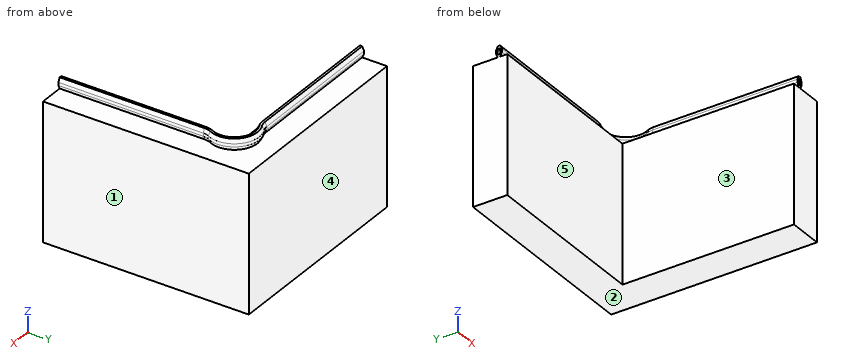
from build123d import *

# Parameters (mm, degrees)
F1_DEPTH = 100


with BuildPart() as f1:
    # F0 (on Top) → F1 (new body)
    with BuildSketch(Plane.XY):
        Polygon((0, -150), (0, 0), (-150, 0), (-150, -25), (-25, -25), (-25, -150), align=None)
    extrude(amount=F1_DEPTH)

    # F4: sweep along a path in F2
    with BuildLine(Plane.XY.offset(100)) as f4_path:
        Line((-150, -18.9), (-44.4089054678, -18.9))
        ThreePointArc((-44.4089054678, -18.9), (-41.6782966505, -18.5851947133), (-39.0909561818, -17.6572959145))
        ThreePointArc((-39.0909561818, -17.6572959145), (-20.6866486348, -20.6866486348), (-17.6572959145, -39.0909561818))
        ThreePointArc((-17.6572959145, -39.0909561818), (-18.5851947133, -41.6782966505), (-18.9, -44.4089054678))
        Line((-18.9, -44.4089054678), (-18.9, -150))
    # F3 (on face) → F4 (sweep)
    with BuildSketch(Plane(origin=(-150, 0, 0), x_dir=(0, -1, 0), z_dir=(-1, 0, 0))):
        Polygon((16.7, 102.875), (18.0713046565, 100), (19.7286953435, 100), (21.1, 102.875), (21.1, 105.075), (19.7286953435, 107.95), (18.0713046565, 107.95), (16.7, 105.075), align=None)
        Polygon((17.75, 104.971631851), (18.2285820574, 105.975), (19.5714179426, 105.975), (20.05, 104.971631851), (20.05, 102.978368149), (19.5714179426, 101.975), (18.2285820574, 101.975), (17.75, 102.978368149), align=None, mode=Mode.SUBTRACT)
    sweep(path=f4_path.line)


solid = f1.part
Work out the finished part from the listing and answer in its coordinate system (mm). Face numbers are marked on the shaded views. A direction names the side the tool comes from. Coordinates: 2 decimals unless noted, no trailing zeros. Write each loop counter-clockwise with the first axis right and the second up, starting at its lowest first coordinate (ties: lowest second). Pieces come first, ordered by that corner, then holes. Notation, with made-up numbers: (6.5, 73.5) - (59.5, 73.5) arc R24 ccw to (59.5, 108.5) - close; hole circle Ø7 at (27, 75). An arc over 180 degrees is marked (long way). One line per question, with ' | ' between items.
1) Find section A-A, the plane y = -69.5. Determine the outline of the cut face in (x, z) (3 decimals).
Checks:
outline: (-25, 0) - (0, 0) - (0, 100) - (-18.071, 100) - (-16.7, 102.875) - (-16.7, 105.075) - (-18.071, 107.95) - (-19.729, 107.95) - (-21.1, 105.075) - (-21.1, 102.875) - (-19.729, 100) - (-25, 100) - close; hole (-20.05, 102.978) - (-19.571, 101.975) - (-18.229, 101.975) - (-17.75, 102.978) - (-17.75, 104.972) - (-18.229, 105.975) - (-19.571, 105.975) - (-20.05, 104.972) - close
2) For the marked faces 4 and 5, determine the directions among +Z, -Z, +X, -X, +Y, -Y from which every point of the face is accessible in a straight line to the end or side of a thin tool.
Checks:
face 4: +Z, -Z, +X, -X, +Y | face 5: +Z, -Z, -X, -Y
3) Find section D-D, the plane x = -9.5. Determine the outline of the cut face in (y, z), and give its area (3 significant figures).
Checks:
outline: (-150, 0) - (0, 0) - (0, 100) - (-150, 100) - close | area: 15,000 mm2
4) Flat-ended cylindrical pins translate along their axes: P1, Ø0.6, axis at y = -98, z = 104, coming from the -X side; P2, Ø2, axis at y = -85, z = 67.5, coming from the -X side; P3, Ø2, axis at x = -128, z = 53.5, coming from the -Y side. Find the tip coordinate at first contact, or state that the pin passes through.
Checks:
P1: x = -21.1 | P2: x = -25 | P3: y = -25
5) The mould has two halves that part along X. Classify the marked faces 1, 2 and 3: +X half, -X half, draft (parallel to the pull), parting line (faces both ways), or undercut.
Checks:
face 1: +X half | face 2: draft | face 3: -X half
6) Consider probe 1 along X at (y, z) = (-121, 77.5); probe 2 along X at (y, z) = (-86, 102.5). Determine where each line is inside the solid, lowest interval first. Write a range as [from, to].
Checks:
probe 1: [-25, 0] | probe 2: [-20.92, -19.82], [-17.98, -16.88]
7) Find section C-C, the plane z = 63. Determine the outline of the cut face in (x, y), and give its area (4 significant figures).
Checks:
outline: (-150, -25) - (-25, -25) - (-25, -150) - (0, -150) - (0, 0) - (-150, 0) - close | area: 6,875 mm2
